Source: CAD feature listing. Evaluate the final solid. Frame: model axes, mm. A direction names the side the tool comes from. Give positions to 0.01 mm unless a question says otherwise; leave off trailing zeros. Order: outer loops, then holes, each group sorted by start corner. A loop starts at its lowest first (then second) coordinate and runs counter-clockwise, first axis right, second up.
from build123d import *

# Parameters (mm, degrees)
F0_W     = 812.8
F0_H     = 152.4
F0_R     = 3.96875
F1_DEPTH = 12.7
F3_DEPTH = 12.7
F5_DEPTH = 12.7
F7_DEPTH = 393.7


with BuildPart() as f1:
    # F0 (on Top) → F1 (new body)
    with BuildSketch(Plane.XY):
        Rectangle(F0_W, F0_H)
        with Locations((-381, -63.5)):
            Circle(F0_R, mode=Mode.SUBTRACT)
        with Locations((-228.6, -63.5)):
            Circle(F0_R, mode=Mode.SUBTRACT)
        with Locations((-76.2, -63.5)):
            Circle(F0_R, mode=Mode.SUBTRACT)
        with Locations((76.2, -63.5)):
            Circle(F0_R, mode=Mode.SUBTRACT)
        with Locations((228.6, -63.5)):
            Circle(F0_R, mode=Mode.SUBTRACT)
        with Locations((381, -63.5)):
            Circle(F0_R, mode=Mode.SUBTRACT)
        with Locations((-381, 63.5)):
            Circle(F0_R, mode=Mode.SUBTRACT)
        with Locations((-228.6, 63.5)):
            Circle(F0_R, mode=Mode.SUBTRACT)
        with Locations((-76.2, 63.5)):
            Circle(F0_R, mode=Mode.SUBTRACT)
        with Locations((76.2, 63.5)):
            Circle(F0_R, mode=Mode.SUBTRACT)
        with Locations((228.6, 63.5)):
            Circle(F0_R, mode=Mode.SUBTRACT)
        with Locations((381, 63.5)):
            Circle(F0_R, mode=Mode.SUBTRACT)
    extrude(amount=F1_DEPTH)

    # F2 (on face) → F3 (join)
    with BuildSketch(Plane(origin=(-406.4, 0, 0), x_dir=(0, -1, 0), z_dir=(-1, 0, 0))):
        Polygon((76.2, 63.5), (-76.2, 63.5), (-76.2, 12.7), (-31.75, 12.7), (-31.75, 50.8), (31.75, 50.8), (31.75, 12.7), (76.2, 12.7), align=None)
    extrude(amount=-F3_DEPTH)

    # F4 (on face) → F5 (join)
    with BuildSketch(Plane.YZ.offset(406.4)):
        Polygon((-76.2, 63.5), (-76.2, 12.7), (-31.75, 12.7), (-31.75, 50.8), (31.75, 50.8), (31.75, 12.7), (76.2, 12.7), (76.2, 63.5), align=None)
    extrude(amount=-F5_DEPTH)

    # F6 (on Right) → F7 (join, symmetric)
    with BuildSketch(Plane.YZ):
        Polygon((69.85, 12.7), (76.2, 12.7), (76.2, 57.15), (71.4375, 57.15), (71.4375, 55.5625), (74.6125, 55.5625), (74.6125, 44.45), (69.85, 44.45), align=None)
        Polygon((-71.4375, 57.15), (-76.2, 57.15), (-76.2, 12.7), (-69.85, 12.7), (-69.85, 44.45), (-74.6125, 44.45), (-74.6125, 55.5625), (-71.4375, 55.5625), align=None)
    extrude(amount=F7_DEPTH, both=True)


solid = f1.part
1) Ray query, L1, parallel to Y at x = 228, z = 7; L2, parallel to Y at x = -76, z = 7; L3, parallel to Y at x = -249.5, z = 48.5. Return the intervals inside material, ascending.
Checks:
L1: y = -76.2 to -67.42, -59.58 to 59.58, 67.42 to 76.2
L2: y = -76.2 to -67.46, -59.54 to 59.54, 67.46 to 76.2
L3: y = -76.2 to -74.61, 74.61 to 76.2
2) First-contact query: pin 1 Ø8 at (x, y) = (-115, 40.5) entering from +Z; pin 2 Ø7 at (x, y) = (228.6, 63.5) entering from -Z. Flat tips, straight axial feed; report the tip coordinate or a pass-through.
Checks:
pin 1: stops at z = 12.7
pin 2: passes through
3) Section query C-C on x = -240.5. Output: boundary loops of the cut face in (y, z), and give its area (3 significant figures).
Checks:
outline: (-76.2, 0) - (76.2, 0) - (76.2, 57.15) - (71.44, 57.15) - (71.44, 55.56) - (74.61, 55.56) - (74.61, 44.45) - (69.85, 44.45) - (69.85, 12.7) - (-69.85, 12.7) - (-69.85, 44.45) - (-74.61, 44.45) - (-74.61, 55.56) - (-71.44, 55.56) - (-71.44, 57.15) - (-76.2, 57.15) - close
area: 2,390 mm2
4) Reachability of faces 5 (the face through (6, -69.85, 28)), 6 (the face through (6, -76.2, 32)), 7 (the face through (400, -31.75, 31)) from +Z, -Z, +X, -X, +Y, -Y: full face, straight path, thin tool, end or side. Return the list, or none.
Checks:
face 5: +Z
face 6: +Z, -Z, +X, -X, -Y
face 7: +X, -X
5) Section query B-B on y = -1. Output: boundary loops of the cut face in (x, z).
Checks:
outline: (-406.4, 0) - (406.4, 0) - (406.4, 12.7) - (-406.4, 12.7) - close; (-406.4, 50.8) - (-393.7, 50.8) - (-393.7, 63.5) - (-406.4, 63.5) - close; (393.7, 50.8) - (406.4, 50.8) - (406.4, 63.5) - (393.7, 63.5) - close
6) Pull-direction query (X, two-part tool) for faces 1 (the face through (-406.4, 1, 53)), 2 (the face through (-6, 69.85, 29)), 3 (the face through (406.4, -1, 53)), 4 (the face through (-400, -1, 63.5)); classes: +X half, -X half, draft (parallel to the pull), parting line (faces both ways), or undercut.
Checks:
face 1: -X half
face 2: undercut
face 3: +X half
face 4: draft
7) Section query D-D on y = 47. Output: boundary loops of the cut face in (x, z).
Checks:
outline: (-406.4, 0) - (406.4, 0) - (406.4, 63.5) - (393.7, 63.5) - (393.7, 12.7) - (-393.7, 12.7) - (-393.7, 63.5) - (-406.4, 63.5) - close
8) Section query A-A on z = 30.5. Output: boundary loops of the cut face in (x, y), and give its area (3 significant figures).
Checks:
outline: (-406.4, -76.2) - (406.4, -76.2) - (406.4, -31.75) - (393.7, -31.75) - (393.7, -69.85) - (-393.7, -69.85) - (-393.7, -31.75) - (-406.4, -31.75) - close; (-406.4, 31.75) - (-393.7, 31.75) - (-393.7, 69.85) - (393.7, 69.85) - (393.7, 31.75) - (406.4, 31.75) - (406.4, 76.2) - (-406.4, 76.2) - close
area: 12,300 mm2
